Check sheet for the modelled part. Datum: model origin and axes. Units: mm. A direction names the side the tool comes from. Round coordinates to 2 decimals unless told otherwise and drop trailing zeros. Write each loop counter-clockwise with the first axis right and the second up, starting at its lowest first coordinate (ties: lowest second). Pieces come first, ordered by that corner, then holes.
Item 1: Cross-section at C-C on x = -7.75. Enter the section's corners in (y, z), plus the area to 3 significant figures.
Item 2: Go/stop test with flat-tipped pins: pin 1 Ø4 at (x, y) = (0, 7.875) entering from -Z; pin 2 Ø4 at (x, y) = (0, -8) entering from +Z. Record where each tip stops, or that it passes through.
Item 3: Material ranges on line 1 (Y direction, x = 0, z = -0.85) (3 decimals); line 2 (Z direction, x = -3.75, y = 8); line 3 (X direction, y = 3, z = -8.75), recorded low to high.
Item 4: Tool access check on faces 5 (the cylindrical face through (5, 0, 1)), 6 (the flat face through (2, -5, -3.75)), 7 (the cylindrical face through (-1.4, 10.66, -1.85)). Record the directions out of +Z, -Z, +X, -X, +Y, -Y that give a thin tool (end or side, any length) a straight path to the whole face; none if there is none.
Item 5: Cross-section at A-A on y = 0. Enter the section's corners in (x, z) (3 decimals).
Item 6: Release check for a two-part mould opening along Y. For faces 1 (the flat face through (2, -5, 0)), 2 (the cylindrical face through (1.08, -4.88, -8.68)), 3 (the cylindrical face through (0.74, -3.32, -6.66)), 4 (the cylindrical face through (-0.33, 6.41, -1.85)) record: +Y half, -Y half, draft (parallel to the pull), parting line (faces both ways), or undercut.
Item 7: Cross-section at D-D on y = -8.75. Enter the section's corners in (x, z) (3 decimals), plus the area to 3 significant figures.
from build123d import *

# Parameters (mm, degrees)
SKETCH3_R                   = 10.75
BOSS_EXTRUDE1_DEPTH         = 3.75
SKETCH4_R                   = 5
BOSS_EXTRUDE2_DEPTH         = 10
BOSS_EXTRUDE3_START         = 1.25
SKETCH5_R                   = 5
BOSS_EXTRUDE3_DEPTH         = 1.25
M8_TAPPED_HOLE1_D           = 6.8
M8_TAPPED_HOLE1_DEPTH       = 15
M8_TAPPED_HOLE1_CSINK_D     = 8.05
M8_TAPPED_HOLE1_CSINK_ANGLE = 90
M8_TAPPED_HOLE1_TIP         = 2.042926105
SKETCH9_R                   = 1.5
CUT_EXTRUDE1_DEPTH          = 3.75


with BuildPart() as part:
    # Sketch3 → Boss-Extrude1 (new body)
    with BuildSketch(Plane.XY):
        Circle(SKETCH3_R)
    extrude(amount=-BOSS_EXTRUDE1_DEPTH)

    # Sketch4 → Boss-Extrude2 (add)
    with BuildSketch(Plane(origin=(0, 0, -3.75), x_dir=(-1, 0, 0), z_dir=(0, 0, -1))):
        Circle(SKETCH4_R)
    extrude(amount=BOSS_EXTRUDE2_DEPTH)

    # Sketch5 → Boss-Extrude3 (add)
    with BuildSketch(Plane.XY.offset(BOSS_EXTRUDE3_START)):
        with Locations(Location((0, 0, 0), (0, 0, 180))):
            Circle(SKETCH5_R)
    extrude(amount=-BOSS_EXTRUDE3_DEPTH)

    # M8 Tapped Hole1
    with Locations(Plane.XY.offset(1.25)):
        with Locations((0, 0)):
            CounterSinkHole(M8_TAPPED_HOLE1_D / 2, M8_TAPPED_HOLE1_CSINK_D / 2, depth=M8_TAPPED_HOLE1_DEPTH, counter_sink_angle=M8_TAPPED_HOLE1_CSINK_ANGLE)
            with Locations((0, 0, -(M8_TAPPED_HOLE1_DEPTH + M8_TAPPED_HOLE1_TIP / 2))):  # 118° drill point
                Cone(0, M8_TAPPED_HOLE1_D / 2, M8_TAPPED_HOLE1_TIP, mode=Mode.SUBTRACT)

    # Sketch9 → Cut-Extrude1 (cut)
    with BuildSketch(Plane.XY):
        with Locations((-7.875, 0)):
            Circle(SKETCH9_R)
        with Locations((0, 7.875)):
            Circle(SKETCH9_R)
        with Locations((7.875, 0)):
            Circle(SKETCH9_R)
        with Locations((0, -7.875)):
            Circle(SKETCH9_R)
    extrude(amount=-CUT_EXTRUDE1_DEPTH, mode=Mode.SUBTRACT)


solid = part.part
Response values:
1. outline: (-7.45, -3.75) - (-1.49, -3.75) - (-1.49, 0) - (-7.45, 0) - close; (1.49, -3.75) - (7.45, -3.75) - (7.45, 0) - (1.49, 0) - close
1. area: 44.7 mm2
2. pin 1: stops at z = -3.75
2. pin 2: stops at z = 0
3. line 1: y = -10.75 to -9.375, -6.375 to -3.4, 3.4 to 6.375, 9.375 to 10.75
3. line 2: z = -3.75 to 0
3. line 3: x = -4 to -1.6, 1.6 to 4
4. face 5: +Z
4. face 6: -Z
4. face 7: +Z, -Z
5. outline: (-10.75, -3.75) - (-9.375, -3.75) - (-9.375, 0) - (-10.75, 0) - close; (-6.375, -3.75) - (-5, -3.75) - (-5, -13.75) - (-3.4, -13.75) - (-3.4, 0.625) - (-4.025, 1.25) - (-5, 1.25) - (-5, 0) - (-6.375, 0) - close; (3.4, -13.75) - (5, -13.75) - (5, -3.75) - (6.375, -3.75) - (6.375, 0) - (5, 0) - (5, 1.25) - (4.025, 1.25) - (3.4, 0.625) - close; (9.375, -3.75) - (10.75, -3.75) - (10.75, 0) - (9.375, 0) - close
6. face 1: draft
6. face 2: parting line
6. face 3: undercut
6. face 4: undercut
7. outline: (-6.245, -3.75) - (-1.218, -3.75) - (-1.218, 0) - (-6.245, 0) - close; (1.218, -3.75) - (6.245, -3.75) - (6.245, 0) - (1.218, 0) - close
7. area: 37.7 mm2
